from build123d import *

# Parameters (mm, degrees)
F1_DEPTH = 40
F2_R     = 5
F2_R_2   = 4.0311299375
F3_DEPTH = 40.001
F5_DEPTH = 10


with BuildPart() as f1:
    # F0 (on Top) → F1 (new body)
    with BuildSketch(Plane.XY):
        Polygon((41.0151937604, 22.0804412934), (-38.9848062396, 22.0804412934), (-38.9848062396, -17.9195587066), (1.0151937604, -17.9195587066), (1.0151937604, -7.9195587066), (41.0151937604, -7.9195587066), align=None)
    extrude(amount=F1_DEPTH)

    # F2 (on face) → F3 (cut, through all)
    with BuildSketch(Plane.XZ.offset(17.9195587066)):
        with BuildLine():
            ThreePointArc((1.0151937604, 10), (22.228397196, 18.7867965644), (31.0151937604, 40))
            ThreePointArc((31.0151937604, 40), (3.5208867316, 69.8951752417), (-28.5662397552, 44.9938753651))
            Line((-28.5662397552, 44.9938753651), (-24.9655683531, 44.9938753651))
            Line((-24.9655683531, 44.9938753651), (-24.9655683531, 40))
            Line((-24.9655683531, 40), (1.0151937604, 40))
            Line((1.0151937604, 40), (1.0151937604, 10))
        make_face()
        with BuildLine():
            ThreePointArc((-24.9655683531, 25), (-13.9848062396, 14.0192378865), (1.0151937604, 10))
            Line((1.0151937604, 10), (1.0151937604, 40))
            Line((1.0151937604, 40), (-24.9655683531, 40))
            Line((-24.9655683531, 40), (-24.9655683531, 25))
        make_face()
        with BuildLine():
            Line((-24.9655683531, 40), (-28.9848062396, 40))
            ThreePointArc((-28.9848062396, 40), (-27.9625810283, 32.2354286469), (-24.9655683531, 25))
            Line((-24.9655683531, 25), (-24.9655683531, 40))
        make_face()
        with Locations((-28.9848062396, 7.9765189439)):
            Circle(F2_R)
        with Locations((31.0151937604, 8.2001261983)):
            Circle(F2_R_2)
        with BuildLine():
            Line((-24.9655683531, 44.9938753651), (-28.5662397552, 44.9938753651))
            ThreePointArc((-28.5662397552, 44.9938753651), (-28.8799814813, 42.5056929712), (-28.9848062396, 40))
            Line((-28.9848062396, 40), (-24.9655683531, 40))
            Line((-24.9655683531, 40), (-24.9655683531, 44.9938753651))
        make_face()
    extrude(amount=-F3_DEPTH, mode=Mode.SUBTRACT)

    # F4 (on face) → F5 (cut)
    with BuildSketch(Plane.XZ.offset(17.9195587066)):
        with BuildLine():
            Line((-19.918359757, 48.6072202153), (-45.8058249796, 48.6072202153))
            Line((-45.8058249796, 48.6072202153), (-45.8058249796, 25))
            Line((-45.8058249796, 25), (-38.9848062396, 25))
            Line((-38.9848062396, 25), (-38.9848062396, 40))
            Line((-38.9848062396, 40), (-28.9848062396, 40))
            ThreePointArc((-28.9848062396, 40), (-27.9625810283, 32.2354286469), (-24.9655683531, 25))
            Line((-24.9655683531, 25), (-19.918359757, 25))
            Line((-19.918359757, 25), (-19.918359757, 48.6072202153))
        make_face()
        with BuildLine():
            Line((-38.9848062396, 40), (-38.9848062396, 25))
            Line((-38.9848062396, 25), (-24.9655683531, 25))
            ThreePointArc((-24.9655683531, 25), (-27.9625810283, 32.2354286469), (-28.9848062396, 40))
            Line((-28.9848062396, 40), (-38.9848062396, 40))
        make_face()
    extrude(amount=-F5_DEPTH, mode=Mode.SUBTRACT)


solid = f1.part
Verification items for the finished model (mm, model axes). A direction names the side the tool comes from. Give positions to 0.01 mm unless a question says otherwise; leave off trailing zeros. Loops run counter-clockwise (first coordinate to the right, second up) from the corner with the lowest first, then second, coordinate; pieces in that order, holes last. Notation, with made-up numbers: (67, 86) - (121, 86) arc R25 ccw to (121, 120) - close; hole circle Ø8 at (-6.75, 15). An arc over 180 degrees is marked (long way). Write item = value, one per line. Start each with the question number.
Q1. Depth check by flat-ended pin: P1, Ø1.5, axis at x = 6, y = 0, coming from the -Z side; P2, Ø11, axis at x = -29.5, y = -14, coming from the +Z side; P3, Ø8, axis at x = 16, z = 6.5, coming from the -Y side; P4, Ø10, axis at x = 14, y = -13.5, coming from the -Z side. Enter the tip coordinate at first touch or a pass-through.
Q2. Mould release check, pull along Z, two halves, no side actions. Record for faces 1 (the face through (-34, -7.92, 33)), 2 (the face through (-24.216, 1.8, 9.478)), 3 (the face through (-32, -13, 25)), 4 (the face through (34.86, 6.87, 9.41)): released by +Z, released by -Z, zero draft, split by the parting line, or undercut.
Q3. Cross-section at D-D, the plane z = 27. Enter the section's corners in (x, y), and give its area (3 significant figures).
Q4. Cross-section at C-C, the plane y = -13. Enter the section's corners in (x, z).
Q5. Tool access check on faces 5 (the face through (1.015, -13, 5)), 6 (the face through (36, 7, 40)). Record the directions out of +Z, -Z, +X, -X, +Y, -Y that give a thin tool (end or side, any length) a straight path to the whole face; none if there is none.
Q6. Thickness scan on line 1 (X direction, y = 17, z = 8); line 2 (Y direction, x = 30, z = 13); line 3 (Z direction, x = -33, y = 15.5). Record the ranges inside material, lowest first.
Q7. Cross-section at A-A, the plane z = 16. Enter the section's corners in (x, y), and give its area (3 significant figures).
Q8. Cross-section at B-B, the plane y = 19.5. Enter the section's corners in (x, z), and give its area (3 significant figures).
Answer key:
q1.P1 = 0
q1.P2 = 25
q1.P3 = -7.92
q1.P4 = through
q2.face_1 = zero draft
q2.face_2 = undercut
q2.face_3 = released by +Z
q2.face_4 = undercut
q3.outline = (-38.98, -7.92) - (-26.02, -7.92) - (-26.02, 22.08) - (-38.98, 22.08) - close; (28.05, -7.92) - (41.02, -7.92) - (41.02, 22.08) - (28.05, 22.08) - close
q3.area = 778 mm^2
q4.outline = (-38.98, 0) - (1.02, 0) - (1.02, 10) arc R30 cw to (-24.97, 25) - (-38.98, 25) - close; hole circle Ø10 at (-28.98, 7.98)
q5.face_5 = +Z, -Z, +X, -Y
q5.face_6 = +Z, +X, -X, +Y, -Y
q6.line_1 = -38.98 to -33.98, -23.98 to 26.99, 35.04 to 41.02
q6.line_2 = -7.92 to 22.08
q6.line_3 = 0 to 5, 10.96 to 40
q7.outline = (-38.98, -17.92) - (-16.98, -17.92) - (-16.98, 22.08) - (-38.98, 22.08) - close; (19.02, -7.92) - (41.02, -7.92) - (41.02, 22.08) - (19.02, 22.08) - close
q7.area = 1,540 mm^2
q8.outline = (-38.98, 0) - (41.02, 0) - (41.02, 40) - (31.02, 40) arc R30 cw to (-28.98, 40) - (-38.98, 40) - close; hole circle Ø10 at (-28.98, 7.98); hole circle Ø8.06 at (31.02, 8.2)
q8.area = 1,660 mm^2
